```python
from build123d import *

# Parameters (mm, degrees)
F1_DEPTH = 5
F2_W     = 635.918021
F2_H     = 207.585454
F3_DEPTH = 25


with BuildPart() as f1:
    # F0 (on Top) → F1 (new body)
    with BuildSketch(Plane.XY):
        Polygon((0, 200), (0, 0), (600, 0), (600, 200), (450, 200), (450, 300), (600, 300), (600, 450), (0, 450), (0, 300), (150, 300), (150, 200), align=None)
        Polygon((600, 0), (0, 0), (150, -200), (450, -200), align=None)
    extrude(amount=F1_DEPTH)

    # F2 (on face) → F3 (cut)
    with BuildSketch(Plane.XY.offset(5)):
        with Locations((317.95901, -103.792727)):
            Rectangle(F2_W, F2_H)
    extrude(amount=-F3_DEPTH, mode=Mode.SUBTRACT)


solid = f1.part
```
For this review, take the finished solid that the model builds, in its own axes (mm). Round coordinates to 2 decimals unless told otherwise and drop trailing zeros. Write each loop counter-clockwise with the first axis right and the second up, starting at its lowest first coordinate (ties: lowest second). Pieces come first, ordered by that corner, then holes. Notation, with made-up numbers: (44.5, -24) -> (101.5, -24) arc R34 cw to (101.5, 7) -> close; hole circle Ø6 at (4.25, -29.5). An arc over 180 degrees is marked (long way). One line per question, with ' | ' between items. Start each with the question number.
1) For pin 1 Ø1.5 at (y, z) = (263, 2) entering from -X, flat-tipped, find the tip position at first contact; note if it passes through.
2) Wall thickness on line 1 along Y through (x, z) = (132, 2.25); line 2 along X through (y, z) = (282.5, 2.6): over which ranges is each line inside the solid? List them lowest first.
3) Add section A-A (x = 97). Write out the cut boundary in (y, z).
4) Add section C-C (y = 239). Write out the cut boundary in (x, z).
5) Add section B-B (z = 3.9). Write out the cut boundary in (x, y).
Reported:
1) pin 1: stops at x = 150
2) line 1: y = 0 to 200, 300 to 450 | line 2: x = 150 to 450
3) outline: (0, 0) -> (200, 0) -> (200, 5) -> (0, 5) -> close; (300, 0) -> (450, 0) -> (450, 5) -> (300, 5) -> close
4) outline: (150, 0) -> (450, 0) -> (450, 5) -> (150, 5) -> close
5) outline: (0, 0) -> (600, 0) -> (600, 200) -> (450, 200) -> (450, 300) -> (600, 300) -> (600, 450) -> (0, 450) -> (0, 300) -> (150, 300) -> (150, 200) -> (0, 200) -> close
